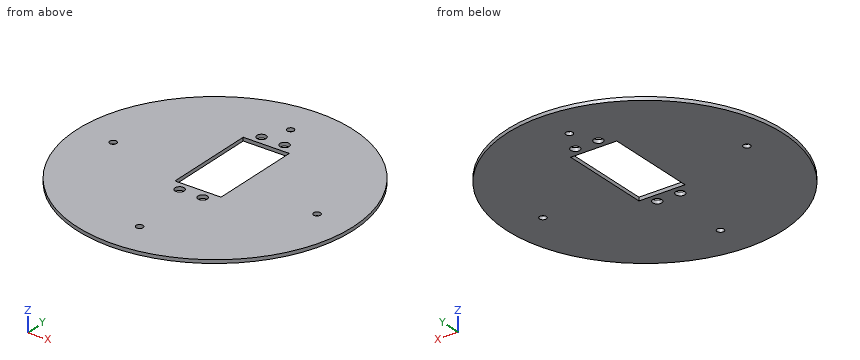
from build123d import *

# Parameters (mm, degrees)
SKETCH_1_R      = 60
SKETCH_1_R_2    = 2
SKETCH_1_R_3    = 1.5
SKETCH_1_W      = 20
SKETCH_1_H      = 40
EXTRUDE_1_DEPTH = 1.5


with BuildPart() as part:
    # 草图1 → 凸台-拉伸1 (new body)
    with BuildSketch(Plane.XY):
        Circle(SKETCH_1_R)
        with Locations((5, 34)):
            Circle(SKETCH_1_R_2, mode=Mode.SUBTRACT)
        with Locations((-5, 34)):
            Circle(SKETCH_1_R_2, mode=Mode.SUBTRACT)
        with Locations((5, -14)):
            Circle(SKETCH_1_R_2, mode=Mode.SUBTRACT)
        with Locations((-5, -14)):
            Circle(SKETCH_1_R_2, mode=Mode.SUBTRACT)
        with Locations((0, 44.25)):
            Circle(SKETCH_1_R_3, mode=Mode.SUBTRACT)
        with Locations((44.25, 0)):
            Circle(SKETCH_1_R_3, mode=Mode.SUBTRACT)
        with Locations((0, -44.25)):
            Circle(SKETCH_1_R_3, mode=Mode.SUBTRACT)
        with Locations((-44.25, 0)):
            Circle(SKETCH_1_R_3, mode=Mode.SUBTRACT)
        with Locations((0, 10)):
            Rectangle(SKETCH_1_W, SKETCH_1_H, mode=Mode.SUBTRACT)
    extrude(amount=EXTRUDE_1_DEPTH)


solid = part.part
Build history of the part. All positions in model axes, mm. Give positions to 0.01 mm unless a question says otherwise; leave off trailing zeros. Write each loop counter-clockwise with the first axis right and the second up, starting at its lowest first coordinate (ties: lowest second). Pieces come first, ordered by that corner, then holes. Notation, with made-up numbers: (-9.5, 73.25) - (28.5, 73.25) arc R38 ccw to (28.5, 112.25) - close; hole circle Ø2 at (86, 72.25). An arc over 180 degrees is marked (long way). Use one line per item in the form item = value. Start each with the question number.
1. Probe line 1 (Y direction, x = 0, z = 0.4); line 2 (Y direction, x = -5, z = 0.3); line 3 (X direction, y = -44.5, z = 0.4). List the from-to ranges inside material, lowest first. Write a range as [from, to].
2. Band-saw the part on D-D on y = -14. Write the cut outline in (x, z), plus the area to 3 significant figures.
3. Band-saw the part on B-B on x = 0. Write the cut outline in (y, z).
4. Band-saw the part on A-A on y = 0. Write the cut outline in (x, z).
5. Drop a flat-ended pin along its axis: pin 1 Ø4.5 at (x, y) = (5, 34) entering from +Z. Give the stop position or say it passes through.
6. Band-saw the part on C-C on z = 0.6. Count the separate pieces of the cut face and the enclosed holes in it, plus the area to 3 significant figures.
Conclusion:
q1.line_1 = [-60, -45.75], [-42.75, -10], [30, 42.75], [45.75, 60]
q1.line_2 = [-59.79, -16], [-12, -10], [30, 32], [36, 59.79]
q1.line_3 = [-40.25, -1.48], [1.48, 40.25]
q2.outline = (-58.34, 0) - (-7, 0) - (-7, 1.5) - (-58.34, 1.5) - close; (-3, 0) - (3, 0) - (3, 1.5) - (-3, 1.5) - close; (7, 0) - (58.34, 0) - (58.34, 1.5) - (7, 1.5) - close
q2.area = 163 mm²
q3.outline = (-60, 0) - (-45.75, 0) - (-45.75, 1.5) - (-60, 1.5) - close; (-42.75, 0) - (-10, 0) - (-10, 1.5) - (-42.75, 1.5) - close; (30, 0) - (42.75, 0) - (42.75, 1.5) - (30, 1.5) - close; (45.75, 0) - (60, 0) - (60, 1.5) - (45.75, 1.5) - close
q4.outline = (-60, 0) - (-45.75, 0) - (-45.75, 1.5) - (-60, 1.5) - close; (-42.75, 0) - (-10, 0) - (-10, 1.5) - (-42.75, 1.5) - close; (10, 0) - (42.75, 0) - (42.75, 1.5) - (10, 1.5) - close; (45.75, 0) - (60, 0) - (60, 1.5) - (45.75, 1.5) - close
q5.pin_1 = 1.5
q6.separate_pieces = 1
q6.enclosed_holes = 9
q6.area = 10,400 mm²
